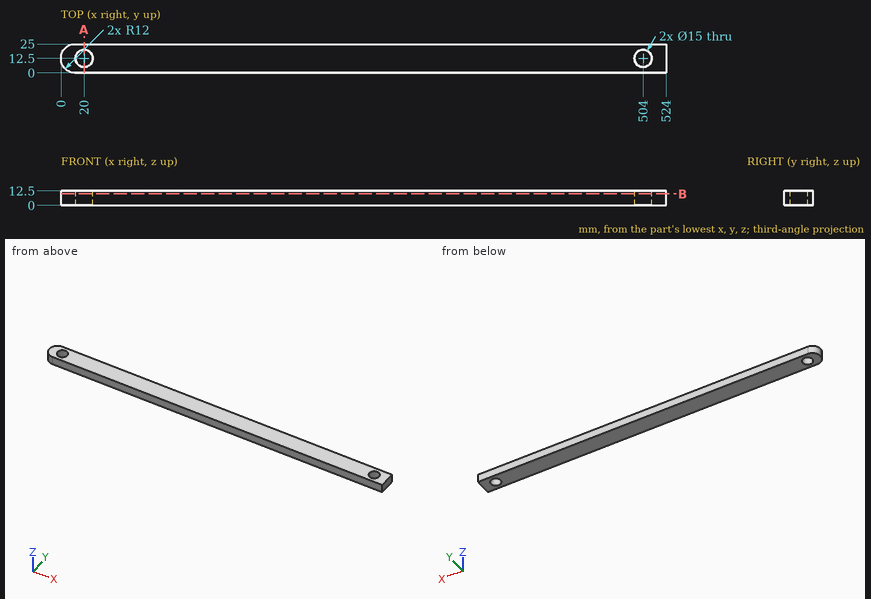
Part print with two shaded views. Sizes in mm from the minimum x, y, z corner. Give positions to 0.01 mm unless a question says otherwise; leave off trailing zeros. Loops run counter-clockwise (first coordinate to the right, second up) from the corner with the lowest first, then second, coordinate; pieces in that order, holes last. Notation, with made-up numbers: (-33, -14.75) -> (-18, -14.75) arc R25 ccw to (-18, 6.25) -> close; hole circle Ø10 at (61, 60). An arc over 180 degrees is marked (long way). One line per question, with ' | ' between items.
Q1. Drop a flat-ended pin along its axis: pin 1 (12 mm diameter, centred on x = 504, y = 12.5, fed in from -Z). Give the stop position or say it passes through.
Filled sheet:
pin 1: passes through
Q2. Cut at A-A, the plane x = 20. Write the cut outline in (y, z), plus the area to 3 significant figures.
Filled sheet:
outline: (0, 0) -> (5, 0) -> (5, 12.5) -> (0, 12.5) -> close; (20, 0) -> (25, 0) -> (25, 12.5) -> (20, 12.5) -> close | area: 125 mm²
Q3. Drill centre lines: line 1 along X through (y, z) = (12.5, 8.5); line 2 along X through (y, z) = (11.5, 7.25); line 3 along Y through (x, z) = (20, 3.5). Where is each one in solid material? Low to high. Write a range as [from, to].
Filled sheet:
line 1: x = [0, 12.5], [27.5, 496.5], [511.5, 524] | line 2: x = [0.01, 12.57], [27.43, 496.57], [511.43, 524] | line 3: y = [0, 5], [20, 25]
Q4. Cut at B-B, the plane z = 10. Write the cut outline in (x, y), plus the area to 3 significant figures.
Filled sheet:
outline: (0, 12) arc R12 ccw to (12, 0) -> (524, 0) -> (524, 25) -> (12, 25) arc R12 ccw to (0, 13) -> close; hole circle Ø15 at (20, 12.5); hole circle Ø15 at (504, 12.5) | area: 12,700 mm²
